Input: part model. Units: mm. Frame: model coordinates. A direction names the side the tool comes from. Give positions to 0.01 mm unless a question says otherwise; leave off trailing zeros. Answer in a Markdown table with one row per item. Add a question column.
1. Access query for faces 5 (the face through (36, 24, 0.66)), 6 (the face through (46, 19, -15)), 7 (the face through (42.58, 31.51, -35.26)). Directions: +Z, -Z, +X, -X, +Y, -Y. A direction counts if a zero-diameter tool reaches every point of the face in a straight line with its end or side. Return the directions, or none.
2. Contact query for flat-ended pins moving along their axis: pin 1 (3 mm diameter, centred on x = 37.5, y = 22, fed in from +Z); pin 2 (12.5 mm diameter, centred on x = 36, y = 8, fed in from -Z); pin 3 (10 mm diameter, centred on x = 14, y = 23, fed in from -Z). Output: stop coordinate, or through.
3. Mould query, pull axis Z, two halves, no side actions, for faces 1 (the face through (24, 31, -19)), 2 (the face through (24, 8, -14)), 3 (the face through (11.38, 28.71, 1.95)), 4 (the face through (12, 24, 0.66)). Classes: released by +Z, released by -Z, zero draft, split by the parting line, or undercut.
4. Section query A-A on x = 4. Count the separate pieces of the cut face and the enclosed holes in it, and give its area (3 significant figures).
5. Ray query, line 1 (X direction, y = 18, z = -15.5); line 2 (Z direction, x = 6, y = 16.5); line 3 (Y direction, x = 10, z = -27). Return the intervals inside material, ascending. Write a range as [from, to].
```python
from build123d import *

# Parameters (mm, degrees)
CROQUIS1_W                        = 48
CROQUIS1_H                        = 32
SALIENTE_EXTRUIR1_DEPTH           = 3.2
CROQUIS2_W                        = 48
CROQUIS2_H                        = 1
SALIENTE_EXTRUIR2_DEPTH           = 39
TALADRO_DE_MARGEN_PARA_M31_D      = 3.2
SALIENTE_EXTRUIR3_DEPTH           = 48
CORTAR_EXTRUIR1_DEPTH             = 46
CORTAR_EXTRUIR2_REACH             = 71.635
CROQUIS7_W                        = 44
CROQUIS7_H                        = 14
SALIENTE_EXTRUIR4_DEPTH           = 2
CORTAR_EXTRUIR3_REACH             = 71.635
CROQUIS9_W                        = 32
CROQUIS9_H                        = 4
CROQUIS10_R                       = 4.75
CORTAR_EXTRUIR4_DEPTH             = 2.54
TALADRO_DE_MARGEN_PARA_M32_REACH  = 69.057
TALADRO_DE_MARGEN_PARA_M32_BORE_R = 1.6


with BuildPart() as part:
    # Croquis1 → Saliente-Extruir1 (new body)
    with BuildSketch(Plane.XY):
        with Locations((24, 16)):
            Rectangle(CROQUIS1_W, CROQUIS1_H)
    extrude(amount=SALIENTE_EXTRUIR1_DEPTH)

    # Croquis2 → Saliente-Extruir2 (add)
    with BuildSketch(Plane(origin=(0, 0, 0), x_dir=(-1, 0, 0), z_dir=(0, 0, -1))):
        with Locations((-24, 31.5)):
            Rectangle(CROQUIS2_W, CROQUIS2_H)
    extrude(amount=SALIENTE_EXTRUIR2_DEPTH)

    # Taladro de margen para M31 (through all)
    with Locations(Plane(origin=(6.5, 32, -18), x_dir=(0, 0, 1), z_dir=(0, 1, 0))):
        with Locations((0, 0), (0, 35)):
            Hole(TALADRO_DE_MARGEN_PARA_M31_D / 2)

    # Croquis5 → Saliente-Extruir3 (add)
    with BuildSketch(Plane.ZY):
        with BuildLine():
            Line((0, 0), (0, 31))
            Line((0, 31), (-39, 31))
            add(Edge.make_bspline(
                [(-39, 31), (-24.225246719, 9.372950474), (0, 0)],
                knots=[0, 0, 0, 1, 1, 1], degree=2))
        make_face()
    extrude(amount=-SALIENTE_EXTRUIR3_DEPTH)

    # Croquis6 → Cortar-Extruir1 (cut)
    with BuildSketch(Plane.ZY):
        with BuildLine():
            Line((0, 31), (-38, 31))
            add(Edge.make_bspline(
                [(-38, 31), (-22.667891875, 11.302250625), (0, 1)],
                knots=[0, 0, 0, 1, 1, 1], degree=2))
            Line((0, 1), (0, 31))
        make_face()
    extrude(amount=-CORTAR_EXTRUIR1_DEPTH, mode=Mode.SUBTRACT)

    # Croquis7 → Cortar-Extruir2 (cut, up to next)
    with BuildSketch(Plane.XZ, mode=Mode.PRIVATE) as cortar_extruir2_sk1:
        with Locations((24, -7)):
            Rectangle(CROQUIS7_W, CROQUIS7_H)
    cortar_extruir2_tool1 = extrude(cortar_extruir2_sk1.sketch, amount=-CORTAR_EXTRUIR2_REACH, mode=Mode.PRIVATE) & part.part
    add(cortar_extruir2_tool1.solids().sort_by_distance((24, 0, -7))[0], mode=Mode.SUBTRACT)

    # Croquis8 → Saliente-Extruir4 (add)
    with BuildSketch(Plane.ZY):
        with BuildLine():
            Line((-38, 31), (0, 31))
            Line((0, 31), (0, 1))
            add(Edge.make_bspline(
                [(-38, 31), (-22.667891875, 11.302250625), (0, 1)],
                knots=[0, 0, 0, 1, 1, 1], degree=2))
        make_face()
    extrude(amount=-SALIENTE_EXTRUIR4_DEPTH)

    # Croquis9 → Cortar-Extruir3 (cut, up to next)
    with BuildSketch(Plane(origin=(0, 32, 0), x_dir=(1, 0, 0), z_dir=(0, 1, 0)), mode=Mode.PRIVATE) as cortar_extruir3_sk1:
        with Locations((24, 34)):
            Rectangle(CROQUIS9_W, CROQUIS9_H)
    cortar_extruir3_tool1 = extrude(cortar_extruir3_sk1.sketch, amount=-CORTAR_EXTRUIR3_REACH, mode=Mode.PRIVATE) & part.part
    add(cortar_extruir3_tool1.solids().sort_by_distance((24, 32, -34))[0], mode=Mode.SUBTRACT)

    # Croquis10 → Cortar-Extruir4 (cut)
    with BuildSketch(Plane.XY.offset(3.2)):
        with Locations((12, 24)):
            Circle(CROQUIS10_R)
        with Locations(Location((36, 24, 0), (0, 0, 180))):
            Circle(CROQUIS10_R)
        with Locations((36, 8)):
            Circle(CROQUIS10_R)
        with Locations(Location((12, 8, 0), (0, 0, 180))):
            Circle(CROQUIS10_R)
    extrude(amount=-CORTAR_EXTRUIR4_DEPTH, mode=Mode.SUBTRACT)

    # Taladro de margen para M32 bore (on position points) → Taladro de margen para M32 (cut, up to next)
    with BuildSketch(Plane(origin=(4, 32, -36), x_dir=(0, 0, 1), z_dir=(0, 1, 0)), mode=Mode.PRIVATE) as taladro_de_margen_para_m32_sk1:
        Circle(TALADRO_DE_MARGEN_PARA_M32_BORE_R)
    taladro_de_margen_para_m32_tool1 = extrude(taladro_de_margen_para_m32_sk1.sketch, amount=-TALADRO_DE_MARGEN_PARA_M32_REACH, mode=Mode.PRIVATE) & part.part
    # Taladro de margen para M32 bore (on position points) → Taladro de margen para M32 (cut, up to next)
    with BuildSketch(Plane(origin=(4, 32, -36), x_dir=(0, 0, 1), z_dir=(0, 1, 0)), mode=Mode.PRIVATE) as taladro_de_margen_para_m32_sk2:
        with Locations((36.2, 0)):
            Circle(TALADRO_DE_MARGEN_PARA_M32_BORE_R)
    taladro_de_margen_para_m32_tool2 = extrude(taladro_de_margen_para_m32_sk2.sketch, amount=-TALADRO_DE_MARGEN_PARA_M32_REACH, mode=Mode.PRIVATE) & part.part
    # Taladro de margen para M32 bore (on position points) → Taladro de margen para M32 (cut, up to next)
    with BuildSketch(Plane(origin=(4, 32, -36), x_dir=(0, 0, 1), z_dir=(0, 1, 0)), mode=Mode.PRIVATE) as taladro_de_margen_para_m32_sk3:
        with Locations((36.2, 40)):
            Circle(TALADRO_DE_MARGEN_PARA_M32_BORE_R)
    taladro_de_margen_para_m32_tool3 = extrude(taladro_de_margen_para_m32_sk3.sketch, amount=-TALADRO_DE_MARGEN_PARA_M32_REACH, mode=Mode.PRIVATE) & part.part
    # Taladro de margen para M32 bore (on position points) → Taladro de margen para M32 (cut, up to next)
    with BuildSketch(Plane(origin=(4, 32, -36), x_dir=(0, 0, 1), z_dir=(0, 1, 0)), mode=Mode.PRIVATE) as taladro_de_margen_para_m32_sk4:
        with Locations((0, 40)):
            Circle(TALADRO_DE_MARGEN_PARA_M32_BORE_R)
    taladro_de_margen_para_m32_tool4 = extrude(taladro_de_margen_para_m32_sk4.sketch, amount=-TALADRO_DE_MARGEN_PARA_M32_REACH, mode=Mode.PRIVATE) & part.part
    add(taladro_de_margen_para_m32_tool1.solids().sort_by_distance((4, 32, -36))[0], mode=Mode.SUBTRACT)
    add(taladro_de_margen_para_m32_tool2.solids().sort_by_distance((4, 32, 0.2))[0], mode=Mode.SUBTRACT)
    add(taladro_de_margen_para_m32_tool3.solids().sort_by_distance((44, 32, 0.2))[0], mode=Mode.SUBTRACT)
    add(taladro_de_margen_para_m32_tool4.solids().sort_by_distance((44, 32, -36))[0], mode=Mode.SUBTRACT)


solid = part.part
```
Answer:
| question | item | result |
|---|---|---|
| 1 | face 5 | +Z |
| 1 | face 6 | none |
| 1 | face 7 | +Y |
| 2 | pin 1 | stops at z = 0.66 |
| 2 | pin 2 | stops at z = -24.06 |
| 2 | pin 3 | stops at z = -36.86 |
| 3 | face 1 | undercut |
| 3 | face 2 | undercut |
| 3 | face 3 | zero draft |
| 3 | face 4 | released by +Z |
| 4 | separate pieces | 3 |
| 4 | enclosed holes | 0 |
| 4 | area | 126 mm² |
| 5 | line 1 | x = [0, 2], [46, 48] |
| 5 | line 2 | z = [-26.59, -24.28], [0, 3.2] |
| 5 | line 3 | y = [16.89, 18.95], [31, 32] |
